Here's how the part is built. I have some questions about the finished solid (model axes, mm). A direction names the side the tool comes from. Give positions to 0.01 mm unless a question says otherwise; leave off trailing zeros. Loops run counter-clockwise (first coordinate to the right, second up) from the corner with the lowest first, then second, coordinate; pieces in that order, holes last. Notation, with made-up numbers: M -27,17.25 L -23,17.25 A26 ccw -23,32.25 Z; hole C 47,57.25 d1. An arc over 180 degrees is marked long. Answer as CSV lines item,"result". Start each with the question number.
Item 1: If I drill on line 1 along Z through (x, y) = (0, -21); line 2 along Y through (x, z) = (26, 15.5), over which ranges is the centre line in solid material (lowest first)? Write a range as from..to.
Item 2: If we mould it in two halves opening along X, with no side actions, what happens to faces 1 (the cylindrical face through (-31.82, -18.8, 24.4)), 2 (the cylindrical face through (41.11, -17.28, -12.95)), 3 (the flat face through (29, -33, 29))? For each: released by +X, released by -X, zero draft, split by the parting line, or undercut.
Item 3: For faces 4 (the flat face through (-1, 0, -1)), 5 (the flat face through (-1, -3, -1)), which set-ups out of +Z, -Z, +X, -X, +Y, -Y let a thin tool reach every point of the face, with its end or its side?
Item 4: I want a section at A-A on x = 0. List the corners of the cut face in (y, z) for me, plus the area to 3 significant figures.
Item 5: Will these pins go through, and if not, where does the flat tip stop? P1, Ø4, axis at y = -23, z = -15, coming from the +X side; P2, Ø1, axis at x = -21, y = -14, coming from the +Z side; P3, Ø2, axis at y = -24.5, z = -11.5, coming from the +X side.
Item 6: I want a section at C-C on z = 0. List the corners of the cut face in (x, y) for me, plus the area to 3 significant figures.
Item 7: I want a section at B-B on y = -15.5. List the corners of the cut face in (x, z) for me, plus the area to 3 significant figures.
from build123d import *

# Parameters (mm, degrees)
SKETCH1_R           = 43.1
SKETCH1_R_2         = 40.1
BOSS_EXTRUDE1_DEPTH = 33
SKETCH1_2_R         = 40.1
BOSS_EXTRUDE2_DEPTH = 3
FILLET1_R           = 2


with BuildPart() as part:
    # Sketch1 → Boss-Extrude1 (new body)
    with BuildSketch(Plane(origin=(0, 0, 0), x_dir=(1, 0, 0), z_dir=(0, 1, 0))):
        Circle(SKETCH1_R)
        Circle(SKETCH1_R_2, mode=Mode.SUBTRACT)
    extrude(amount=-BOSS_EXTRUDE1_DEPTH)

    # Sketch1<2> → Boss-Extrude2 (add)
    with BuildSketch(Plane(origin=(0, 0, 0), x_dir=(1, 0, 0), z_dir=(0, 1, 0))):
        Circle(SKETCH1_2_R)
    extrude(amount=-BOSS_EXTRUDE2_DEPTH)

    # Fillet1
    fillet1_edges = [part.edges().sort_by_distance(p)[0] for p in [
        (-43.1, 0, 0),
        (-40.1, -3, 0),
    ]]
    fillet(fillet1_edges, radius=FILLET1_R)


solid = part.part
Result:
1,line 1,"-43.1..-40.1, 40.1..43.1"
1,line 2,"-3..0"
2,face 1,"undercut"
2,face 2,"split by the parting line"
2,face 3,"zero draft"
3,face 4,"+Z, -Z, +X, -X, +Y"
3,face 5,"-Y"
4,outline,"M -33,-43.1 L -2,-43.1 A2 ccw 0,-41.1 L 0,41.1 A2 ccw -2,43.1 L -33,43.1 L -33,40.1 L -5,40.1 A2 cw -3,38.1 L -3,-38.1 A2 cw -5,-40.1 L -33,-40.1 Z"
4,area,"439 mm^2"
5,P1,"x = 41.09"
5,P2,"z = 37.91"
5,P3,"x = 41.8"
6,outline,"M -43.1,-33 L -40.1,-33 L -40.1,-5 A2 cw -38.1,-3 L 38.1,-3 A2 cw 40.1,-5 L 40.1,-33 L 43.1,-33 L 43.1,-2 A2 ccw 41.1,0 L -41.1,0 A2 ccw -43.1,-2 Z"
6,area,"439 mm^2"
7,outline,"C 0,0 d86.2; hole C 0,0 d80.2"
7,area,"784 mm^2"
